Here's the drawing with two shaded views (mm, measured from the low corner). I have some questions. A direction names the side the tool comes from. Give positions to 0.01 mm unless a question says otherwise; leave off trailing zeros. Order: outer loops, then holes, each group sorted by start corner. A loop starts at its lowest first (then second) coordinate and runs counter-clockwise, first axis right, second up. Notation, with made-up numbers: M 13,18 L 44,18 A19 ccw 44,23 Z; hole C 80,-13.5 d1. An arc over 180 degrees is marked long. One line per question, with ' | ' between items. Start each with the question number.
1) Please list where these lines run through material, in increasing order: line 1 along Z through (x, y) = (34.55, 19.25); line 2 along X through (y, z) = (22.5, 6.5); line 3 along Z through (x, y) = (34.7, 6.75). Write a range as [from, to].
2) If we section it at C-C, the plane z = 30.5: Please give me the cut outline in (x, y).
3) If we section it at B-B, the plane y = 6.75: Please give me the cut outline in (x, z).
4) For the marked faces 5 and 6, which set-ups out of +Z, -Z, +X, -X, +Y, -Y let a thin tool reach every point of the face, with its end or its side?
5) I'm going to push flat-ended pins straight in: pin 1 Ø9.5 at (x, z) = (12, 24) entering from +Y; pin 2 Ø3.5 at (y, z) = (19.25, 30.5) entering from +X. Where does each tip first touch, or does it pass through?
6) If we section it at A-A, the plane z = 18: Please give me the cut outline in (x, y).
7) Thinking about a two-plate mould opening in X: for the marked faces 1, 2, 3 and 4, which applies, +X half, -X half, draft (parallel to the pull), parting line (faces both ways), or undercut?
8) If we section it at D-D, the plane x = 31: Please give me the cut outline in (y, z).
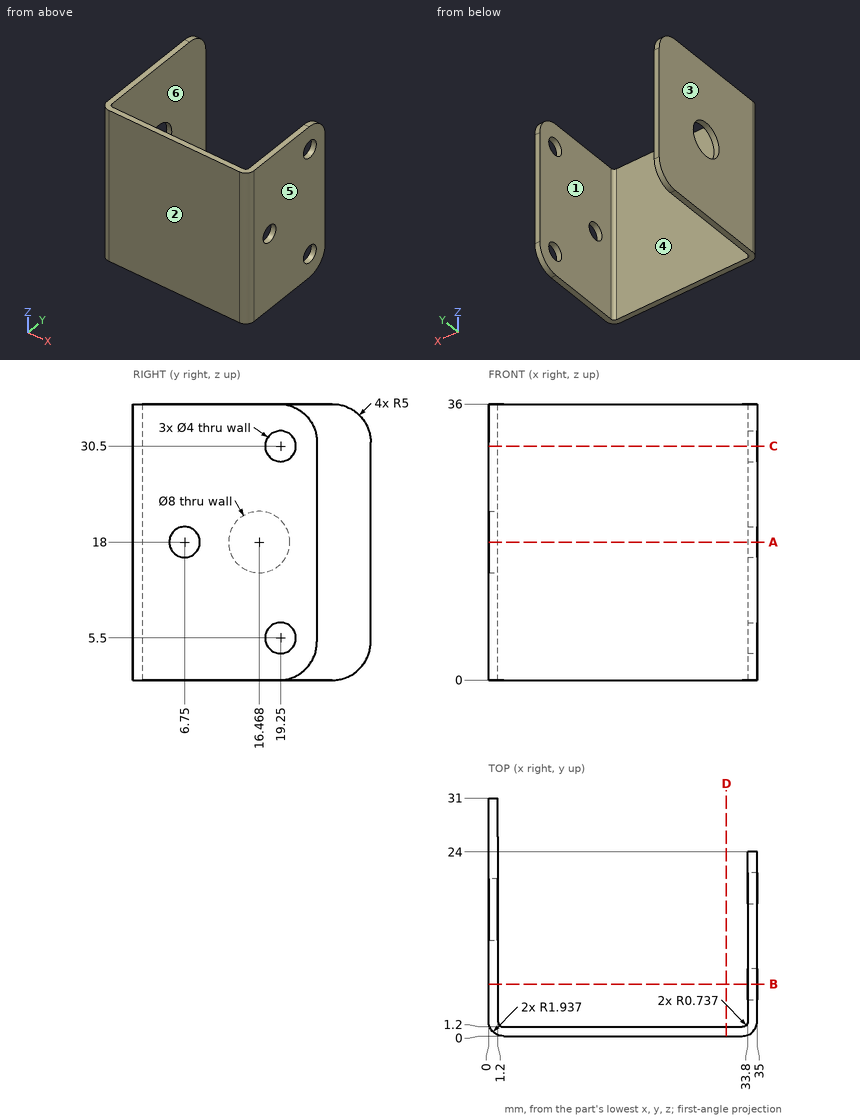
Results found:
1) line 1: z = [0.01, 3.5], [7.5, 28.5], [32.5, 35.99] | line 2: x = [0, 1.2], [33.8, 35] | line 3: z = [0, 16], [20, 36]
2) outline: M 0,1.94 A1.94 ccw 1.94,0 L 33.06,0 A1.94 ccw 35,1.94 L 35,17.25 L 33.8,17.25 L 33.8,1.94 A0.74 cw 33.06,1.2 L 1.94,1.2 A0.74 cw 1.2,1.94 L 1.2,31 L 0,31 Z; M 33.8,21.25 L 35,21.25 L 35,24 L 33.8,24 Z
3) outline: M 0,0 L 1.2,0 L 1.2,36 L 0,36 Z; M 33.8,0 L 35,0 L 35,16 L 33.8,16 Z; M 33.8,20 L 35,20 L 35,36 L 33.8,36 Z
4) face 5: +Z, -Z, +X, +Y, -Y | face 6: +Z, -Z, +Y
5) pin 1: stops at y = 1.2 | pin 2: stops at x = 1.2
6) outline: M 0,1.94 A1.94 ccw 1.94,0 L 33.06,0 A1.94 ccw 35,1.94 L 35,4.75 L 33.8,4.75 L 33.8,1.94 A0.74 cw 33.06,1.2 L 1.94,1.2 A0.74 cw 1.2,1.94 L 1.2,12.47 L 0,12.47 Z; M 0,20.47 L 1.2,20.47 L 1.2,31 L 0,31 Z; M 33.8,8.75 L 35,8.75 L 35,24 L 33.8,24 Z
7) face 1: undercut | face 2: draft | face 3: -X half | face 4: undercut
8) outline: M 0,0 L 1.2,0 L 1.2,36 L 0,36 Z
